Source: three-view drawing plus pictorial views. Frame: mm from the lowest corner of the part. A direction names the side the tool comes from. Give positions to 0.01 mm unless a question says otherwise; leave off trailing zeros. Loops run counter-clockwise (first coordinate to the right, second up) from the corner with the lowest first, then second, coordinate; pieces in that order, holes last.
1. Material intervals for line 1 along Z through (x, y) = (8, 1.5); line 2 along Y through (x, z) = (32, 27.5); line 3 along Z through (x, y) = (52.5, 5.5), sorted ascending.
2. Draft query along Z for the marked faces 1, 2 and 3. Return one class per face: +Z half, -Z half, draft (parallel to the pull), parting line (faces both ways), or undercut.
3. Section B-B, the plane z = 26. Output: boundary loops of the cut face in (x, y), then the cut area to 3 significant figures.
4. First-contact query: P1, Ø3.5, axis at y = 7, z = 5.5, coming from the +X side; P2, Ø1.6, axis at y = 4, z = 28, coming from the +X side; P3, Ø2.5, axis at x = 52, y = 6.5, coming from the +Z side. Flat tips, straight axial feed; report the tip coordinate or a pass-through.
5. Section D-D, the plane y = 2. Output: boundary loops of the cut face in (x, z).
6. Section A-A, the plane y = 8.25. Output: boundary loops of the cut face in (x, z), then the cut area to 3 significant figures.
7. Section C-C, the plane x = 50. Output: boundary loops of the cut face in (y, z), then the cut area to 4 significant figures.
8. Access query for the marked faces 4, 5, 6 and 7. Directions: +Z, -Z, +X, -X, +Y, -Y. A direction counts if a zero-diameter tool reaches every point of the face in a straight line with its end or side. Return the directions, or none.
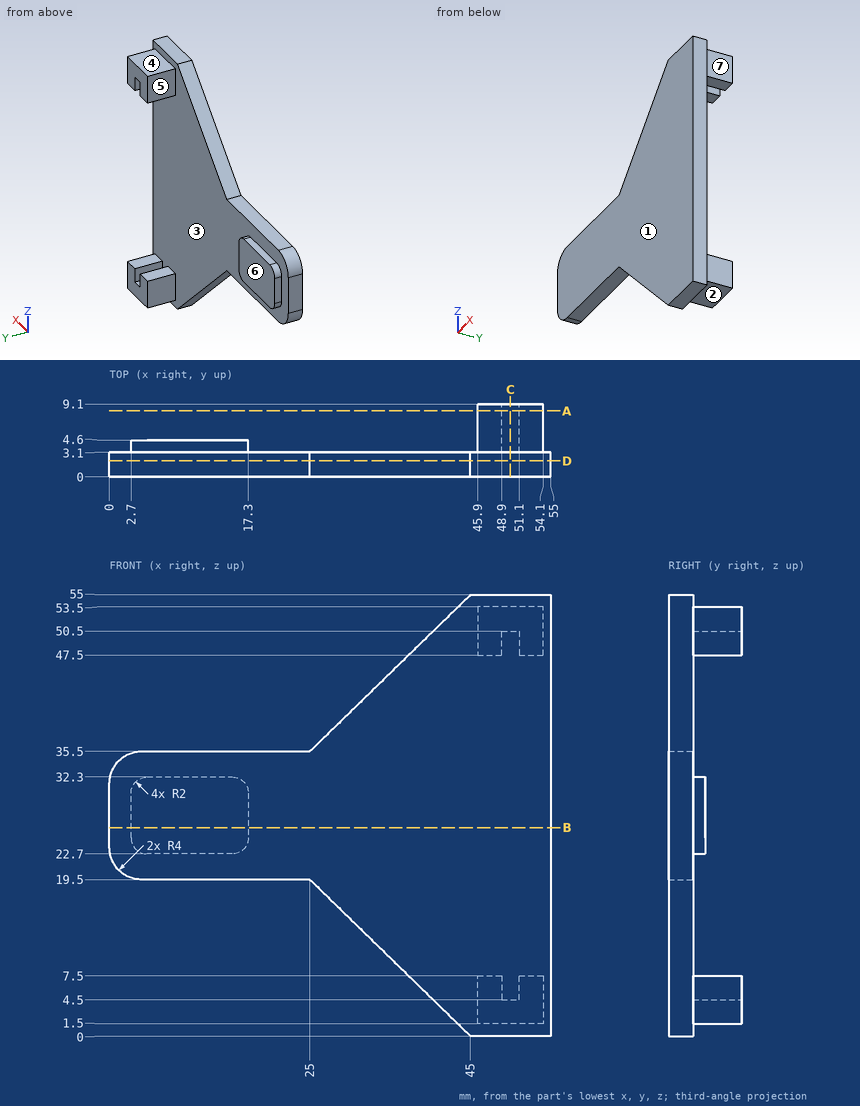
Answers below:
1. line 1: z = 19.5 to 35.5
1. line 2: y = 0 to 3.1
1. line 3: z = 1.5 to 7.5, 47.5 to 53.5
2. face 1: draft
2. face 2: -Z half
2. face 3: undercut
3. outline: (0, 0) - (55, 0) - (55, 3.1) - (17.3, 3.1) - (17.3, 4.6) - (2.7, 4.6) - (2.7, 3.1) - (0, 3.1) - close
3. area: 192 mm2
4. P1: stops at x = 54.1
4. P2: stops at x = 17.3
4. P3: stops at z = 53.5
5. outline: (0, 23.5) arc R4 ccw to (4, 19.5) - (25, 19.5) - (45, 0) - (55, 0) - (55, 55) - (45, 55) - (25, 35.5) - (4, 35.5) arc R4 ccw to (0, 31.5) - close
6. outline: (45.9, 1.5) - (54.1, 1.5) - (54.1, 7.5) - (51.1, 7.5) - (51.1, 4.5) - (48.9, 4.5) - (48.9, 7.5) - (45.9, 7.5) - close; (45.9, 47.5) - (48.9, 47.5) - (48.9, 50.5) - (51.1, 50.5) - (51.1, 47.5) - (54.1, 47.5) - (54.1, 53.5) - (45.9, 53.5) - close
6. area: 85.2 mm2
7. outline: (0, 0) - (3.1, 0) - (3.1, 1.5) - (9.1, 1.5) - (9.1, 4.5) - (3.1, 4.5) - (3.1, 50.5) - (9.1, 50.5) - (9.1, 53.5) - (3.1, 53.5) - (3.1, 55) - (0, 55) - close
7. area: 206.5 mm2
8. face 4: +Z, +X, -X, +Y
8. face 5: +Z, -Z, -X, +Y
8. face 6: +Z, -Z, +X, -X, +Y
8. face 7: +Z, -Z, +X, +Y
